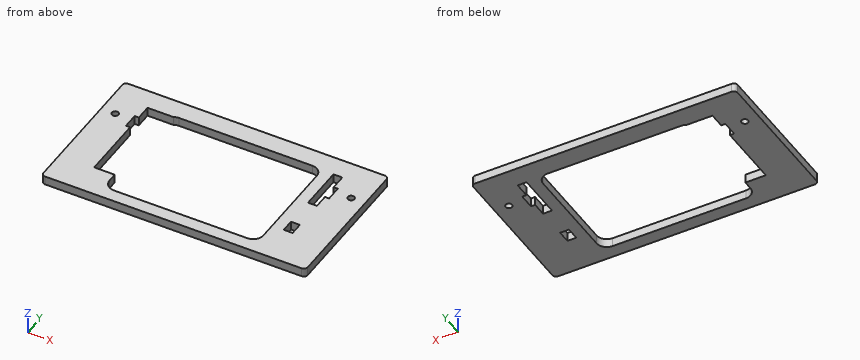
from build123d import *

# Parameters (mm, degrees)
SKETCH1_W           = 206
SKETCH1_H           = 114.5
BOSS_EXTRUDE1_DEPTH = 6.9
SKETCH2_W           = 120
SKETCH2_H           = 88
CUT_EXTRUDE1_DEPTH  = 119.043095944
FILLET1_R           = 8
SKETCH7_R           = 2.54
CUT_EXTRUDE5_DEPTH  = 119.043095944
SKETCH9_W           = 6.96
SKETCH9_H           = 35
SKETCH9_H_2         = 10
CUT_EXTRUDE7_DEPTH  = 119.043095944
SKETCH11_W          = 3.25
SKETCH11_H          = 12
CUT_EXTRUDE8_DEPTH  = 119.043095944
FILLET2_R           = 3
SKETCH8_R           = 1.775
CUT_EXTRUDE6_DEPTH  = 119.043095944
SKETCH10_W          = 6.8
SKETCH10_H          = 3
BOSS_EXTRUDE3_DEPTH = 6.9
FILLET3_R           = 1.5
CUT_EXTRUDE9_DEPTH  = 120.526869364
CUT_EXTRUDE10_DEPTH = 119.043095944
SKETCH15_R          = 1.775
BOSS_EXTRUDE4_DEPTH = 6.9


with BuildPart() as part:
    # Sketch1 → Boss-Extrude1 (new body)
    with BuildSketch(Plane.XY):
        Rectangle(SKETCH1_W, SKETCH1_H)
    extrude(amount=-BOSS_EXTRUDE1_DEPTH)

    # Sketch2 → Cut-Extrude1 (cut, through all)
    with BuildSketch(Plane.XY):
        with Locations((0, -1.75)):
            Rectangle(SKETCH2_W, SKETCH2_H)
    extrude(amount=-CUT_EXTRUDE1_DEPTH, mode=Mode.SUBTRACT)

    # Fillet1
    fillet1_edges = [part.edges().sort_by_distance(p)[0] for p in [
        (-60, -45.75, -3.45),
        (-60, 42.25, -3.45),
        (60, 42.25, -3.45),
        (60, -45.75, -3.45),
    ]]
    fillet(fillet1_edges, radius=FILLET1_R)

    # Sketch7 → Cut-Extrude5 (cut, through all)
    with BuildSketch(Plane.XY):
        with Locations((-92, 25)):
            Circle(SKETCH7_R)
    cut_extrude5 = extrude(amount=-CUT_EXTRUDE5_DEPTH, mode=Mode.SUBTRACT)

    # Sketch9 → Cut-Extrude7 (cut, through all)
    with BuildSketch(Plane.XY):
        with Locations((-72.5, 23.75)):
            Rectangle(SKETCH9_W, SKETCH9_H)
        with Locations((-72.5, -22.25)):
            Rectangle(SKETCH9_W, SKETCH9_H_2)
    cut_extrude7 = extrude(amount=-CUT_EXTRUDE7_DEPTH, mode=Mode.SUBTRACT)

    # Sketch11 → Cut-Extrude8 (cut, through all)
    with BuildSketch(Plane.XY):
        with Locations((-77.605, 23.25)):
            Rectangle(SKETCH11_W, SKETCH11_H)
    cut_extrude8 = extrude(amount=-CUT_EXTRUDE8_DEPTH, mode=Mode.SUBTRACT)

    # Mirror2: Cut-Extrude5, Cut-Extrude7, Cut-Extrude8 across plane
    add(cut_extrude5.mirror(Plane(origin=(0, 0, 0), x_dir=(0, 0, 1), z_dir=(1, 0, 0))), mode=Mode.SUBTRACT)
    add(cut_extrude7.mirror(Plane(origin=(0, 0, 0), x_dir=(0, 0, 1), z_dir=(1, 0, 0))), mode=Mode.SUBTRACT)
    add(cut_extrude8.mirror(Plane(origin=(0, 0, 0), x_dir=(0, 0, 1), z_dir=(1, 0, 0))), mode=Mode.SUBTRACT)

    # Fillet2
    fillet2_edges = [part.edges().sort_by_distance(p)[0] for p in [
        (-103, 57.25, -3.45),
        (103, 57.25, -3.45),
        (103, -57.25, -3.45),
        (-103, -57.25, -3.45),
    ]]
    fillet(fillet2_edges, radius=FILLET2_R)

    # Sketch8 → Cut-Extrude6 (cut, through all)
    with BuildSketch(Plane.XY):
        with Locations((72, -36.75)):
            Circle(SKETCH8_R)
        with Locations((-72, -36.75)):
            Circle(SKETCH8_R)
    extrude(amount=-CUT_EXTRUDE6_DEPTH, mode=Mode.SUBTRACT)

    # Sketch10 → Boss-Extrude3 (add)
    with BuildSketch(Plane.XY):
        with Locations((-38.4, -58.75)):
            Rectangle(SKETCH10_W, SKETCH10_H)
        with Locations((38.4, -58.75)):
            Rectangle(SKETCH10_W, SKETCH10_H)
    extrude(amount=-BOSS_EXTRUDE3_DEPTH)

    # Fillet3
    fillet3_edges = [part.edges().sort_by_distance(p)[0] for p in [
        (-35, -60.25, -3.45),
        (-41.8, -60.25, -3.45),
        (35, -60.25, -3.45),
        (41.8, -60.25, -3.45),
    ]]
    fillet(fillet3_edges, radius=FILLET3_R)

    # Sketch13 → Cut-Extrude9 (cut, through all)
    with BuildSketch(Plane.XY):
        with BuildLine():
            Line((-40.3, -60.25), (-36.5, -60.25))
            ThreePointArc((-36.5, -60.25), (-35.439339828, -59.810660172), (-35, -58.75))
            Line((-35, -58.75), (-35, -57.25))
            Line((-35, -57.25), (-41.8, -57.25))
            Line((-41.8, -57.25), (-41.8, -58.75))
            ThreePointArc((-41.8, -58.75), (-41.360660172, -59.810660172), (-40.3, -60.25))
        make_face()
        with BuildLine():
            Line((35, -57.25), (35, -58.75))
            ThreePointArc((35, -58.75), (35.439339828, -59.810660172), (36.5, -60.25))
            Line((36.5, -60.25), (40.3, -60.25))
            ThreePointArc((40.3, -60.25), (41.360660172, -59.810660172), (41.8, -58.75))
            Line((41.8, -58.75), (41.8, -57.25))
            Line((41.8, -57.25), (35, -57.25))
        make_face()
        with BuildLine():
            Line((-60, -37.75), (-60, -39.25))
            ThreePointArc((-60, -39.25), (-57.656854249, -44.906854249), (-52, -47.25))
            Line((-52, -47.25), (52, -47.25))
            ThreePointArc((52, -47.25), (57.656854249, -44.906854249), (60, -39.25))
            Line((60, -39.25), (60, -37.75))
            ThreePointArc((60, -37.75), (57.656854249, -43.406854249), (52, -45.75))
            Line((52, -45.75), (-52, -45.75))
            ThreePointArc((-52, -45.75), (-57.656854249, -43.406854249), (-60, -37.75))
        make_face()
    extrude(amount=-CUT_EXTRUDE9_DEPTH, mode=Mode.SUBTRACT)

    # Sketch14 → Cut-Extrude10 (cut, through all)
    with BuildSketch(Plane.XY):
        Polygon((-69.02, 6.25), (-75.98, 6.25), (-75.98, -32.25), (-60, -32.25), (-60, 34.25), (-60, 41.25), (-69.02, 41.25), align=None)
        with BuildLine():
            Line((-55.872983346, 41.25), (-60, 41.25))
            Line((-60, 41.25), (-60, 34.25))
            ThreePointArc((-60, 34.25), (-58.891439137, 38.313012013), (-55.872983346, 41.25))
        make_face()
    extrude(amount=-CUT_EXTRUDE10_DEPTH, mode=Mode.SUBTRACT)

    # Sketch15 → Boss-Extrude4 (add)
    with BuildSketch(Plane.XY):
        with Locations((72, -36.75)):
            Circle(SKETCH15_R)
        with Locations((-72, -36.75)):
            Circle(SKETCH15_R)
    extrude(amount=-BOSS_EXTRUDE4_DEPTH)


solid = part.part
Source: CAD feature listing. Evaluate the final solid. Frame: model axes, mm. Round coordinates to 2 decimals unless told otherwise and drop trailing zeros. Write each loop counter-clockwise with the first axis right and the second up, starting at its lowest first coordinate (ties: lowest second). Pieces come first, ordered by that corner, then holes. Notation, with made-up numbers: M -7,21 L -1,21 A21 cw -1,47 Z; hole C -31.5,-18 d4. An arc over 180 degrees is marked long. One line per item, written item: value. Start each with the question number.
Item 1: Section query B-B (y = -30). Return the cut outline in (x, z).
Item 2: Ray query, L1, parallel to Y at x = 74.5, z = -4; L2, parallel to X at y = 22, z = -2; L3, parallel to X at y = -20, z = -5.5. Return the intervals inside material, ascending. Write a range as from..to.
Item 3: Section query A-A (x = 32). Return the cut outline in (y, z), plus the area to 4 significant figures.
Item 4: Section query D-D (z = -1.75). State how many separate pieces and enclosed holes the cut face has, plus the area to 3 significant figures.
Item 5: Section query C-C (y = 12). Return the cut outline in (x, z).
Result set:
1. outline: M -103,-6.9 L -75.98,-6.9 L -75.98,0 L -103,0 Z; M 60,-6.9 L 103,-6.9 L 103,0 L 60,0 Z
2. L1: y = -57.25..-27.25, -17.25..6.25, 41.25..57.25
2. L2: x = -103..-79.23, 60..69.02, 79.23..103
2. L3: x = -103..-75.98, 60..69.02, 75.98..103
3. outline: M -57.25,-6.9 L -47.25,-6.9 L -47.25,0 L -57.25,0 Z; M 42.25,-6.9 L 57.25,-6.9 L 57.25,0 L 42.25,0 Z
3. area: 172.5 mm²
4. separate pieces: 1
4. enclosed holes: 5
4. area: 11,300 mm²
5. outline: M -103,-6.9 L -75.98,-6.9 L -75.98,0 L -103,0 Z; M 60,-6.9 L 69.02,-6.9 L 69.02,0 L 60,0 Z; M 75.98,-6.9 L 103,-6.9 L 103,0 L 75.98,0 Z
